```python
from build123d import *

# Parameters (mm, degrees)
F1_DEPTH = 32.5
F2_DEPTH = 65
F3_DEPTH = 32.5


# Not quite as in the source:
# - a feature names something its author has since deleted; it is built from what else it names


with BuildPart() as f1:
    # F0 (on Front) → F1 (new body, symmetric)
    with BuildSketch(Plane.XZ):
        with BuildLine():
            Line((1900, 0), (0, 0))
            Line((0, 0), (0, -1200))
            Line((0, -1200), (1600, -1200))
            ThreePointArc((1600, -1200), (1953.5533905933, -1053.5533905933), (2100, -700))
            Line((2100, -700), (2100, -200))
            ThreePointArc((2100, -200), (2041.4213562373, -58.5786437627), (1900, 0))
        make_face()
    extrude(amount=F1_DEPTH, both=True)

    # F0 (on Front) → F2 (join)
    with BuildSketch(Plane.XZ):
        with BuildLine():
            Line((-20, -1220), (1600, -1220))
            ThreePointArc((1600, -1220), (1967.695526217, -1067.695526217), (2120, -700))
            Line((2120, -700), (2120, -200))
            ThreePointArc((2120, -200), (2055.563491861, -44.436508139), (1900, 20))
            Line((1900, 20), (-20, 20))
            Line((-20, 20), (-20, -1220))
        make_face()
        with BuildLine():
            Line((0, -1200), (0, 0))
            Line((0, 0), (1900, 0))
            ThreePointArc((1900, 0), (2041.4213562373, -58.5786437627), (2100, -200))
            Line((2100, -200), (2100, -700))
            ThreePointArc((2100, -700), (1953.5533905933, -1053.5533905933), (1600, -1200))
            Line((1600, -1200), (0, -1200))
        make_face(mode=Mode.SUBTRACT)
    extrude(amount=-F2_DEPTH)

    # F0 (on Front) → F3 (join)
    with BuildSketch(Plane.XZ):
        with BuildLine():
            Line((-20, -1220), (1600, -1220))
            ThreePointArc((1600, -1220), (1967.695526217, -1067.695526217), (2120, -700))
            Line((2120, -700), (2120, -200))
            ThreePointArc((2120, -200), (2055.563491861, -44.436508139), (1900, 20))
            Line((1900, 20), (-20, 20))
            Line((-20, 20), (-20, -1220))
        make_face()
        with BuildLine():
            Line((0, -1200), (0, 0))
            Line((0, 0), (1900, 0))
            ThreePointArc((1900, 0), (2041.4213562373, -58.5786437627), (2100, -200))
            Line((2100, -200), (2100, -700))
            ThreePointArc((2100, -700), (1953.5533905933, -1053.5533905933), (1600, -1200))
            Line((1600, -1200), (0, -1200))
        make_face(mode=Mode.SUBTRACT)
    extrude(amount=F3_DEPTH)


solid = f1.part
```
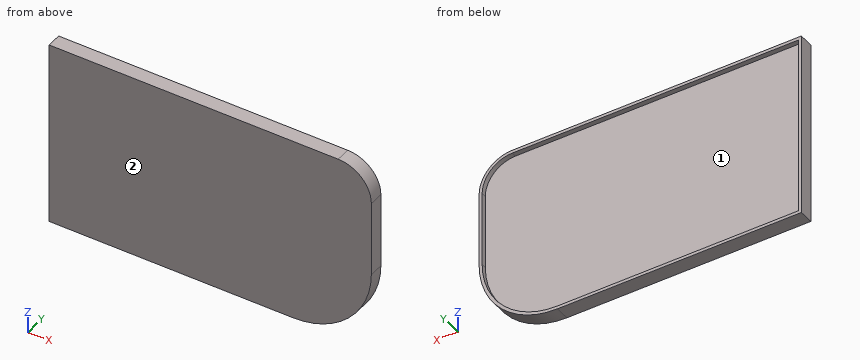
Here's how the part is built. I have some questions about the finished solid (model axes, mm). Face numbers are marked on the shaded views. A direction names the side the tool comes from. Round coordinates to 2 decimals unless told otherwise and drop trailing zeros. Loops run counter-clockwise (first coordinate to the right, second up) from the corner with the lowest first, then second, coordinate; pieces in that order, holes last.
1. Suppose I cut it at B-B, the plane z = -680. Please give me the cut outline in (x, y), and give its area (3 significant figures).
Answers:
outline: (-20, -32.5) - (2120, -32.5) - (2120, 65) - (2100, 65) - (2100, 32.5) - (0, 32.5) - (0, 65) - (-20, 65) - close
area: 140,000 mm2
2. If I drill on probe 1 along X at (y, z) = (45, -495.5); probe 2 along Y at (x, z) = (331, -312); probe 3 along Z at (x, y) = (516, 49), over which ranges is the centre line in solid material (lowest first)?
Answers:
probe 1: x = -20 to 0, 2100 to 2120
probe 2: y = -32.5 to 32.5
probe 3: z = -1220 to -1200, 0 to 20
3. For the marked faces 1 and 2, which set-ups out of +Z, -Z, +X, -X, +Y, -Y let a thin tool reach every point of the face, with its end or its side?
Answers:
face 1: +Y
face 2: +Z, -Z, +X, -X, -Y
4. Suppose I cut it at C-C, the plane y = 47.5. Please give me the cut outline in (x, z), and give its area (3 significant figures).
Answers:
outline: (-20, -1220) - (1600, -1220) arc R520 ccw to (2120, -700) - (2120, -200) arc R220 ccw to (1900, 20) - (-20, 20) - close; hole (0, -1200) - (1600, -1200) arc R500 ccw to (2100, -700) - (2100, -200) arc R200 ccw to (1900, 0) - (0, 0) - close
area: 127,000 mm2
5. Suppose I cut it at A-A, the plane x = 1483. Please give me the cut outline in (y, z).
Answers:
outline: (-32.5, -1220) - (65, -1220) - (65, -1200) - (32.5, -1200) - (32.5, 0) - (65, 0) - (65, 20) - (-32.5, 20) - close
6. Will this pin go through, and if not, where does the flat tip stop? pin 1 (1.5 mm diameter, centred on x = 1435, z = -238.5, fed in from +Y).
Answers:
pin 1: stops at y = 32.5
